Autodesk Inventor part; units mm, degrees
ref_plane "YZ Plane" through (0, 0, 0) normal (1, 0, 0) x (0, 1, 0)
ref_plane "XZ Plane" through (0, 0, 0) normal (0, 1, 0) x (-1, 0, 0)
ref_plane "XY Plane" through (0, 0, 0) normal (0, 0, 1) x (1, 0, 0)
sketch "Sketch1" plane through (0, 0, 0) normal (0, 1, 0) x (-1, 0, 0)
  line L0 (0, 0) -> (110, 0)
  line L1 (110, 0) -> (110, -110)
  line L2 (110, -110) -> (0, -110)
  line L3 (0, -110) -> (0, 0)
  circle A0 centre (5, -5) radius 2.75
  line L4 (55, 0) -> (55, -110) construction
  line L5 (0, -55) -> (110, -55) construction
  circle A1 centre (5, -105) radius 2.75
  circle A2 centre (105, -5) radius 2.75
  circle A3 centre (105, -105) radius 2.75
  dimension "d0" = 110
  dimension "d1" = 110
  dimension "d2" = 5.5
  dimension "d5" = 100
  dimension "d8" = 100
  dimension "d11" = 5
  dimension "d12" = 5
extrude "Extrusion1" add sketch "Sketch1" along normal blind 6
sketch "Sketch2" plane through (0, 6, 0) normal (0, 1, 0) x (1, 0, 0)
  line L0 (0, 0) -> (0, 110) construction
  line L1 (0, 55) -> (-110, 55) construction
  line L2 (-110, 110) -> (-110, 0) construction
  line L3 (-110, 0) -> (0, 0) construction
  line L4 (-55, 0) -> (-55, 110) construction
  line L5 (0, 110) -> (-110, 110) construction
  circle A0 centre (-20, 55) radius 1.65
  circle A1 centre (-55, 55) radius 1.65
  circle A2 centre (-90, 55) radius 1.65
  point P0 (-110, 7.25)
  point P1 (-2.25, 110)
  dimension "d18" = 3.3
  dimension "d22" = 20
  dimension "d36" = 35
extrude "Extrusion2" cut sketch "Sketch2" against normal blind 6
thread "Thread1"
thread "Thread2"
thread "Thread3"
properties part number "Deska izolovaná" material "PC/ABS Plastic"
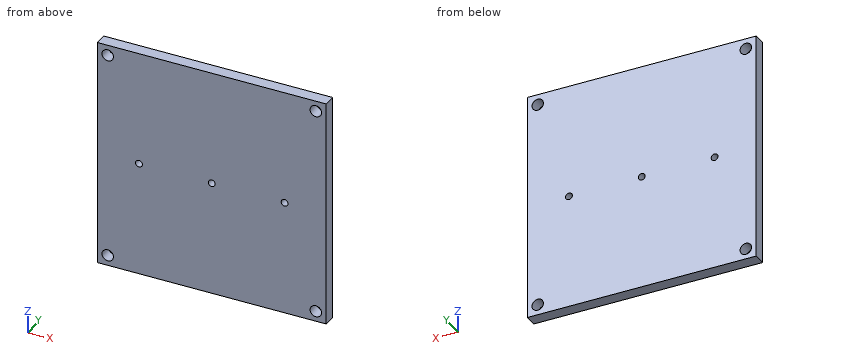
CAD build for the part. Positions are in the model's coordinates, mm. Round coordinates to 2 decimals unless told otherwise and drop trailing zeros. Write each loop counter-clockwise with the first axis right and the second up, starting at its lowest first coordinate (ties: lowest second). Pieces come first, ordered by that corner, then holes. Notation, with made-up numbers: (85.25, 29) -> (102.25, 29) arc R29 ccw to (102.25, 68) -> close; hole circle Ø1 at (72.5, 11.25). An arc over 180 degrees is marked (long way). Answer in a Markdown table with one row per item. Add a question column.
Item 1: Drop a flat-ended pin along its axis: pin 1 Ø3.5 at (x, z) = (-5, -5) entering from -Y. Give the stop position or say it passes through.
Item 2: Saw through at A-A, the plane z = -5. Write the cut outline in (x, y), then the cut area to 3 significant figures.
Item 3: Saw through at B-B, the plane x = -5. Write the cut outline in (y, z).
Item 4: Drill centre lines: line 1 (Z direction, x = -5, y = 1.65); line 2 (X direction, y = 1.45, z = -55); line 3 (Z direction, x = -90, y = 3.6). Where is each one in solid material? Low to high. Write a range as from..to.
Item 5: Saw through at C-C, the plane x = -90. Write the cut outline in (y, z), then the cut area to 3 significant figures.
Findings below:
| question | item | result |
|---|---|---|
| 1 | pin 1 | passes through |
| 2 | outline | (-110, 0) -> (-107.75, 0) -> (-107.75, 6) -> (-110, 6) -> close; (-102.25, 0) -> (-7.75, 0) -> (-7.75, 6) -> (-102.25, 6) -> close; (-2.25, 0) -> (0, 0) -> (0, 6) -> (-2.25, 6) -> close |
| 2 | area | 594 mm^2 |
| 3 | outline | (0, -110) -> (6, -110) -> (6, -107.75) -> (0, -107.75) -> close; (0, -102.25) -> (6, -102.25) -> (6, -7.75) -> (0, -7.75) -> close; (0, -2.25) -> (6, -2.25) -> (6, 0) -> (0, 0) -> close |
| 4 | line 1 | z = -110..-107.75, -102.25..-7.75, -2.25..0 |
| 4 | line 2 | x = -110..-91.65, -88.35..-56.65, -53.35..-21.65, -18.35..0 |
| 4 | line 3 | z = -110..-56.65, -53.35..0 |
| 5 | outline | (0, -110) -> (6, -110) -> (6, -56.65) -> (0, -56.65) -> close; (0, -53.35) -> (6, -53.35) -> (6, 0) -> (0, 0) -> close |
| 5 | area | 640 mm^2 |
